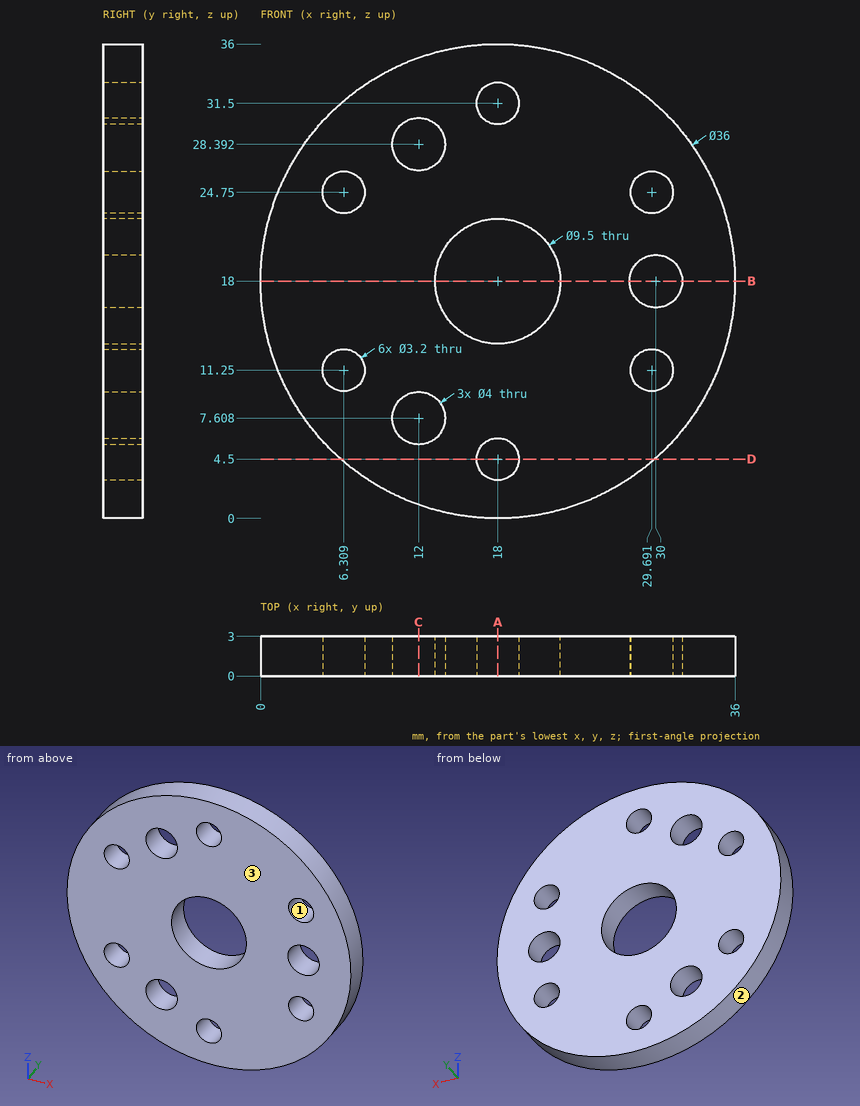
Could you check a few things on this drawing? It's one solid part, dimensions in mm from its lowest x, y, z. Coordinates: 2 decimals unless noted, no trailing zeros. Order: outer loops, then holes, each group sorted by start corner. A loop starts at its lowest first (then second) coordinate and runs counter-clockwise, first axis right, second up. Notation, with made-up numbers: (9.5, 46.5) - (35.5, 46.5) arc R26 ccw to (35.5, 65.5) - close; hole circle Ø9 at (68, 3.5). An arc over 180 degrees is marked (long way). One line per question, with ' | ' between items. Start each with the question number.
1. Please list where these lines run through material, in increasing order: line 1 along X through (y, z) = (1.65, 18); line 2 along X through (y, z) = (1.3, 11.25); line 3 along Z through (x, y) = (7, 2.4). Write a range as [from, to].
2. I'm going to push flat-ended pins straight in: pin 1 Ø6 at (x, z) = (31, 17) entering from -Y; pin 2 Ø1 at (y, z) = (0.5, 8) entering from +X. Where does each tip first touch, or does it pass through?
3. If we mould it in two halves opening along Z, with no side actions, what happens to the marked faces 1, 2 and 3? For each: released by +Z, released by -Z, zero draft, split by the parting line, or undercut.
4. If we section it at C-C (x = 12): Write out the boundary of the cut face in (y, z).
5. If we section it at A-A (x = 18): Write out the boundary of the cut face in (y, z).
6. If we section it at B-B (z = 18): Write out the boundary of the cut face in (x, y), and give its area (3 significant figures).
7. If we section it at D-D (z = 4.5): Write out the boundary of the cut face in (x, y).
Model answer:
1) line 1: x = [0, 13.25], [22.75, 28], [32, 36] | line 2: x = [1.31, 4.71], [7.91, 28.09], [31.29, 34.69] | line 3: z = [3.75, 9.81], [12.69, 23.31], [26.19, 32.25]
2) pin 1: stops at y = 0 | pin 2: stops at x = 33.29
3) face 1: undercut | face 2: split by the parting line | face 3: zero draft
4) outline: (0, 1.03) - (3, 1.03) - (3, 5.61) - (0, 5.61) - close; (0, 9.61) - (3, 9.61) - (3, 26.39) - (0, 26.39) - close; (0, 30.39) - (3, 30.39) - (3, 34.97) - (0, 34.97) - close
5) outline: (0, 0) - (3, 0) - (3, 2.9) - (0, 2.9) - close; (0, 6.1) - (3, 6.1) - (3, 13.25) - (0, 13.25) - close; (0, 22.75) - (3, 22.75) - (3, 29.9) - (0, 29.9) - close; (0, 33.1) - (3, 33.1) - (3, 36) - (0, 36) - close
6) outline: (0, 0) - (13.25, 0) - (13.25, 3) - (0, 3) - close; (22.75, 0) - (28, 0) - (28, 3) - (22.75, 3) - close; (32, 0) - (36, 0) - (36, 3) - (32, 3) - close | area: 67.5 mm²
7) outline: (6.09, 0) - (16.4, 0) - (16.4, 3) - (6.09, 3) - close; (19.6, 0) - (29.91, 0) - (29.91, 3) - (19.6, 3) - close
